Model file for the job. Use its own axes, mm. Face numbers are marked on the shaded views. A direction names the side the tool comes from. Give positions to 0.01 mm unless a question says otherwise; leave off trailing zeros. Order: outer loops, then holes, each group sorted by start corner. A loop starts at its lowest first (then second) coordinate and runs counter-clockwise, first axis right, second up. Notation, with made-up numbers: M 19,50 L 70,50 A20 cw 70,77 Z; hole C 82,10 d8. An arc over 180 degrees is marked long. Return JSON: item names as keys, results as strings. Group by question number.
1. Slice it at D-D on x = -18. List the corners of the cut face in (y, z).
2. 3-axis set-ups, long thin cutter, end or side, ignore diameter. For the marked faces 1 and 2: which of +Z, -Z, +X, -X, +Y, -Y reach the whole face in a straight line?
3. Slice it at B-B on y = 5. List the corners of the cut face in (x, z), then the cut area to 3 significant figures.
4. Slice it at A-A on x = 25. List the corners of the cut face in (y, z).
5. Wall check: probe 1 along Y at (x, z) = (18, 7.55); probe 2 along Y at (x, z) = (-1, 7.25); probe 3 along Y at (x, z) = (-41, 9.75). Give the ranges that are in metal, low to high. Write a range as [from, to].
6. Pin check, flat tips, straight feed: pin 1 (6.5 mm diameter, centred on x = -41, y = -10, fed in from +Z); pin 2 (2.5 mm diameter, centred on x = 30.5, z = 8.5, fed in from +Y); pin 3 (3.5 mm diameter, centred on x = 14.35, y = 53.1, fed in from +Z); pin 4 (5 mm diameter, centred on y = 42, z = 9, fed in from +X). Stop position of each tip, or through.
7. Slice it at C-C on y = -10. List the corners of the cut face in (x, z), then the cut area to 3 significant figures.
8. Two-plate mould, pull along X, no slides. Class the marked faces 3 and 4: released by +X, released by -X, zero draft, split by the parting line, or undercut.
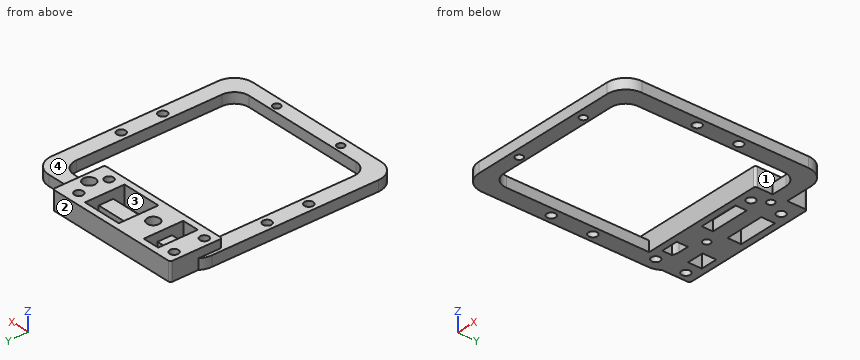
from build123d import *

# Parameters (mm, degrees)
SKETCH002_R      = 1.8
SKETCH002_R_2    = 2.1
SKETCH002_R_3    = 2.458824
EXTRUDE001_DEPTH = 5
SKETCH006_R      = 2.1
SKETCH006_R_2    = 3
SKETCH006_W      = 19
SKETCH006_H      = 19.003748
SKETCH006_W_2    = 8.15
SKETCH006_H_2    = 19
EXTRUDE005_DEPTH = 9


with BuildPart() as pair_connector_extrude:
    # Sketch002 → Extrude001 (new body)
    with BuildSketch(Plane.XY):
        with BuildLine():
            Line((-36, -49), (0, -49))
            Line((0, -49), (36, -49))
            ThreePointArc((36, -49), (42.363961, -46.363961), (45, -40))
            Line((45, -40), (45, 0))
            Line((45, 0), (45, 40))
            ThreePointArc((45, 40), (42.363961, 46.363961), (36, 49))
            Line((36, 49), (0, 49))
            Line((0, 49), (-36, 49))
            ThreePointArc((-36, 49), (-42.363961, 46.363961), (-45, 40))
            Line((-45, 40), (-45, 0))
            Line((-45, 0), (-45, -40))
            ThreePointArc((-45, -40), (-42.363961, -46.363961), (-36, -49))
        make_face()
        with Locations((-18, 45)):
            Circle(SKETCH002_R, mode=Mode.SUBTRACT)
        with Locations((18, 45)):
            Circle(SKETCH002_R, mode=Mode.SUBTRACT)
        with Locations((-18, -45)):
            Circle(SKETCH002_R, mode=Mode.SUBTRACT)
        with Locations((18, -45)):
            Circle(SKETCH002_R, mode=Mode.SUBTRACT)
        with Locations((-41, 10)):
            Circle(SKETCH002_R_2, mode=Mode.SUBTRACT)
        with Locations((-41, -10)):
            Circle(SKETCH002_R_2, mode=Mode.SUBTRACT)
        with Locations((-39.177948, 38.628017)):
            Circle(SKETCH002_R_3, mode=Mode.SUBTRACT)
        with Locations((41, -10)):
            Circle(SKETCH002_R_2, mode=Mode.SUBTRACT)
        with Locations((41, 10)):
            Circle(SKETCH002_R_2, mode=Mode.SUBTRACT)
        with BuildLine():
            Line((-30, -42), (0, -42))
            Line((0, -42), (30, -42))
            ThreePointArc((30, -42), (34.949747, -39.949747), (37, -35))
            Line((37, -35), (37, 0))
            Line((37, 0), (37, 35))
            ThreePointArc((37, 35), (34.949747, 39.949747), (30, 42))
            Line((30, 42), (0, 42))
            Line((0, 42), (-30, 42))
            ThreePointArc((-30, 42), (-34.949747, 39.949747), (-37, 35))
            Line((-37, 35), (-37, 0))
            Line((-37, 0), (-37, -35))
            ThreePointArc((-37, -35), (-34.949747, -39.949747), (-30, -42))
        make_face(mode=Mode.SUBTRACT)
    extrude(amount=EXTRUDE001_DEPTH)


with BuildPart() as pair_connector_extrude_1:
    # Extrude001 placement: moved
    add(pair_connector_extrude.part.moved(Location((0, 0, 6.2))))


with BuildPart() as pair_connector_fusion:
    # Sketch006 → Extrude005 (new body)
    with BuildSketch(Plane.XY):
        with BuildLine():
            Line((-42.4, 58.6), (21.6, 58.6))
            ThreePointArc((22.6, 57.6), (22.307107, 58.307107), (21.6, 58.6))
            Line((22.6, 57.6), (22.6, 34.6))
            ThreePointArc((21.596193, 33.596252), (22.305988, 33.890222), (22.6, 34.6))
            Line((-42.4, 33.6), (21.596193, 33.596252))
            ThreePointArc((-43.4, 34.6), (-43.10709, 33.89291), (-42.4, 33.6))
            Line((-43.4, 34.6), (-43.401347, 57.598594))
            ThreePointArc((-42.4, 58.6), (-43.10808, 58.306691), (-43.401347, 57.598594))
        make_face()
        with Locations((-39.15, 53.1)):
            Circle(SKETCH006_R, mode=Mode.SUBTRACT)
        with Locations((14.35, 53.1)):
            Circle(SKETCH006_R, mode=Mode.SUBTRACT)
        with Locations((-39.15, 38.6)):
            Circle(SKETCH006_R, mode=Mode.SUBTRACT)
        with Locations((14.35, 38.6)):
            Circle(SKETCH006_R, mode=Mode.SUBTRACT)
        with Locations((18, 45)):
            Circle(SKETCH006_R_2, mode=Mode.SUBTRACT)
        with Locations((-18, 45)):
            Circle(SKETCH006_R_2, mode=Mode.SUBTRACT)
        with Locations((-1.5, 46.098126)):
            Rectangle(SKETCH006_W, SKETCH006_H, mode=Mode.SUBTRACT)
        with Locations((-29.075, 46.1)):
            Rectangle(SKETCH006_W_2, SKETCH006_H_2, mode=Mode.SUBTRACT)
    extrude(amount=EXTRUDE005_DEPTH)


with BuildPart() as pair_connector_fusion_1:
    # Extrude005 placement: moved
    add(pair_connector_fusion.part.moved(Location((0, 0, 6.2))))

    # Fusion008: union pair connector extrude
    add(pair_connector_extrude_1.part)


solid = pair_connector_fusion_1.part
Result:
{
 "1": {"outline": "M -49,6.2 L -46.8,6.2 L -46.8,11.2 L -49,11.2 Z; M -43.2,6.2 L -42,6.2 L -42,11.2 L -43.2,11.2 Z; M 33.6,6.2 L 43.2,6.2 L 43.2,11.2 L 42,11.2 L 42,15.2 L 33.6,15.2 Z; M 46.8,6.2 L 58.6,6.2 L 58.6,15.2 L 48,15.2 L 48,11.2 L 46.8,11.2 Z"},
 "2": {"face 1": "+Z", "face 2": "+Z, -Z, +X, -X, +Y"},
 "3": {"outline": "M -45,6.2 L -37,6.2 L -37,11.2 L -45,11.2 Z; M 37,6.2 L 45,6.2 L 45,11.2 L 37,11.2 Z", "area": "80.0 mm2"},
 "4": {"outline": "M -49,6.2 L -42,6.2 L -42,11.2 L -49,11.2 Z; M 42,6.2 L 49,6.2 L 49,11.2 L 42,11.2 Z"},
 "5": {"probe 1": "y = [-49, -46.8], [-43.2, -42], [33.6, 43.2], [46.8, 58.6]", "probe 2": "y = [-49, -42], [33.6, 36.6], [42, 49], [55.6, 58.6]", "probe 3": "y = [-47.48, -12.1], [-7.9, 7.9], [12.1, 37.61], [39.59, 52.11], [54.09, 58.6]"},
 "6": {"pin 1": "stops at z = 11.2", "pin 2": "stops at y = 49", "pin 3": "passes through", "pin 4": "stops at x = 45"},
 "7": {"outline": "M -45,6.2 L -43.1,6.2 L -43.1,11.2 L -45,11.2 Z; M -38.9,6.2 L -37,6.2 L -37,11.2 L -38.9,11.2 Z; M 37,6.2 L 38.9,6.2 L 38.9,11.2 L 37,11.2 Z; M 43.1,6.2 L 45,6.2 L 45,11.2 L 43.1,11.2 Z", "area": "38.0 mm2"},
 "8": {"face 3": "undercut", "face 4": "zero draft"}
}
